```python
from build123d import *

# Parameters (mm, degrees)
SKETCH_1_R          = 2.5
EXTRUDE_1_DEPTH     = 2.5
SKETCH_2_OUTSIDE_W  = 70.512
SKETCH_2_OUTSIDE_H  = 33.683
CUT_EXTRUDE_1_DEPTH = 5


with BuildPart() as part:
    # 草圖1 → 填料-伸長1 (new body, symmetric)
    with BuildSketch(Plane.XY):
        with BuildLine():
            Line((45.485924683, 14.569854348), (-1.018385662, 4.895190563))
            ThreePointArc((-1.018385662, 4.895190563), (-4.973728622, -0.511882402), (0, -5))
            Line((0, -5), (29, -5))
            ThreePointArc((29, -5), (30.248921949, -4.841507406), (31.418665946, -4.376077586))
            Line((31.418665946, -4.376077586), (48.922976291, 5.298586199))
            ThreePointArc((48.922976291, 5.298586199), (51.192518904, 11.412680042), (45.485924683, 14.569854348))
        make_face()
        with Locations((46.504310345, 9.674663785)):
            Circle(SKETCH_1_R, mode=Mode.SUBTRACT)
        with Locations((29, 0)):
            Circle(SKETCH_1_R, mode=Mode.SUBTRACT)
        Circle(SKETCH_1_R, mode=Mode.SUBTRACT)
    extrude(amount=EXTRUDE_1_DEPTH, both=True)

    # 草圖2 outside → 除料-伸長1 (cut)
    with BuildSketch(Plane.XY.offset(2.5)):
        with Locations((23.252, 4.8375)):
            Rectangle(SKETCH_2_OUTSIDE_W, SKETCH_2_OUTSIDE_H)
        with BuildLine():
            ThreePointArc((45.79340971, 4.725459779), (50.890857954, 12.074288771), (41.953237231, 11.745348096))
            ThreePointArc((41.953237231, 11.745348096), (36.933542301, 6.318443182), (29.667856416, 4.955196041))
            ThreePointArc((29.667856416, 4.955196041), (28.134691665, 4.924554953), (26.682918959, 4.43070372))
            ThreePointArc((26.682918959, 4.43070372), (14.5, 1.437415904), (2.317081041, 4.43070372))
            ThreePointArc((2.317081041, 4.43070372), (-4.999984203, 0.012568795), (2.294776385, -4.442296855))
            ThreePointArc((2.294776385, -4.442296855), (14.5, -1.476041996), (26.705223615, -4.442296855))
            ThreePointArc((26.705223615, -4.442296855), (30.657237876, -4.717368188), (33.568899121, -2.031049192))
            ThreePointArc((33.568899121, -2.031049192), (38.547411457, 3.398479533), (45.79340971, 4.725459779))
        make_face(mode=Mode.SUBTRACT)
    extrude(amount=-CUT_EXTRUDE_1_DEPTH, mode=Mode.SUBTRACT)


solid = part.part
```
The model under review builds one solid part; all positions refer to its coordinate system, in mm. Round coordinates to 2 decimals unless told otherwise and drop trailing zeros. Order: outer loops, then holes, each group sorted by start corner. A loop starts at its lowest first (then second) coordinate and runs counter-clockwise, first axis right, second up. Notation, with made-up numbers: M 56,88.5 L 96,88.5 A22 cw 96,102.5 Z; hole C -5.5,-20 d9. An arc over 180 degrees is marked long. Use a Markdown table: item, result.
1) Consider section D-D (x = 12.5). Write out the cut boundary in (y, z), then the cut area to 3 significant figures.
Report:
| item | result |
|---|---|
| outline | M -1.55,-2.5 L 1.51,-2.5 L 1.51,2.5 L -1.55,2.5 Z |
| area | 15.3 mm^2 |
2) Consider section C-C (y = 0). Write out the cut boundary in (x, z), then the cut area to 3 significant figures.
Report:
| item | result |
|---|---|
| outline | M -5,-2.5 L -2.5,-2.5 L -2.5,2.5 L -5,2.5 Z; M 2.5,-2.5 L 26.5,-2.5 L 26.5,2.5 L 2.5,2.5 Z; M 31.5,-2.5 L 34.73,-2.5 L 34.73,2.5 L 31.5,2.5 Z |
| area | 149 mm^2 |
3) Insertion check: pin 1 (4.5 mm diameter, centred on x = 46.5, y = 9.67, fed in from -Z); pin 2 (6.5 mm diameter, centred on x = 0, y = 0, fed in from -Z); pin 3 (1 mm diameter, centred on y = 3.5, z = -0.5, fed in from +X); pin 4 (3 mm diameter, centred on x = 11, z = -1, fed in from +Y). Each pin has a flat end and moves straight along its axis. Give the tip position at first contact, or say it passes through.
Report:
| item | result |
|---|---|
| pin 1 | through |
| pin 2 | z = -2.5 |
| pin 3 | x = 39.81 |
| pin 4 | y = 1.92 |
4) Consider section A-A (y = 11.25). Write out the cut boundary in (x, z), then the cut area to 3 significant figures.
Report:
| item | result |
|---|---|
| outline | M 41.71,-2.5 L 44.56,-2.5 L 44.56,2.5 L 41.71,2.5 Z; M 48.45,-2.5 L 51.25,-2.5 L 51.25,2.5 L 48.45,2.5 Z |
| area | 28.3 mm^2 |
5) Wall thickness on line 1 along Y through (x, z) = (0, -0.5); line 2 along X through (y, z) = (1, 1.95); line 3 along X through (y, z) = (-0.75, 1.95): over which ranges is each line inside the solid? List them lowest first. Write a range as [from, to].
Report:
| item | result |
|---|---|
| line 1 | [-5, -2.5], [2.5, 5] |
| line 2 | [-4.9, -2.29], [2.29, 26.71], [31.29, 35.53] |
| line 3 | [-4.94, -2.38], [2.38, 26.62], [31.38, 34.24] |
6) Consider section B-B (z = 1.05). Write out the cut boundary in (x, y).
Report:
| item | result |
|---|---|
| outline | M 2.29,-4.44 A26.59 cw 26.71,-4.44 A5 ccw 33.57,-2.03 A11.58 cw 45.79,4.73 A5 ccw long 41.95,11.75 A11.77 cw 29.67,4.96 A5 ccw 26.68,4.43 A26.29 cw 2.32,4.43 A5 ccw long Z; hole C 0,0 d5; hole C 29,0 d5; hole C 46.5,9.67 d5 |
7) Draft analysis for pull direction X (two halves, no side actions). For faces 1 (the face through (37.025, 6.37, 0.035)), 2 (the face through (23, 2, 2.5)), state which applies: released by +X, released by -X, zero draft, split by the parting line, or undercut.
Report:
| item | result |
|---|---|
| face 1 | undercut |
| face 2 | zero draft |
